Answer from the drawing. Dimensions are ordinates in mm from the lowest x, y and z of the part. A direction names the side the tool comes from. Give positions to 0.01 mm unless a question says otherwise; leave off trailing zeros. Loops run counter-clockwise (first coordinate to the right, second up) from the corner with the lowest first, then second, coordinate; pieces in that order, holes last. Notation, with made-up numbers: (35, 29) - (41, 29) arc R8 ccw to (41, 38) - close; hole circle Ø11 at (74.25, -18). An arc over 180 degrees is marked (long way). One line per question, with ' | ' between items. Start each with the question number.
1. Section C-C (x = 5) is taken. Determine the outline of the cut face in (y, z), plus the area to 4 significant figures.
2. For a pull along X with two mould halves and no side action, classify the marked faces 3, 4 and 5 as released by +X, released by -X, zero draft, split by the parting line, or undercut.
3. Section D-D (x = 7.75) is taken. Determine the outline of the cut face in (y, z).
4. Which of the six approach directions +Z, -Z, +X, -X, +Y, -Y give full straight-line access (tool end or side, diameter ignored) to the marked faces 1 and 2?
5. Each of these flat-tipped pins is pushed along its axis until it touches: pin 1 (1 mm diameter, centred on x = 7.5, z = 0.5, fed in from -Y); pin 2 (1.2 mm diameter, centred on x = 4.5, z = 1, fed in from -Y). Where does it stop, or does it pass through?
6. Section A-A (y = 3.25) is taken. Determine the outline of the cut face in (x, z).
7. Find the intervals of material crossed by line 1 (X direction, y = 3.75, z = 2.05); line 2 (Y direction, x = 3.25, z = 2.1); line 3 (Y direction, x = 9.25, z = 2.2), in increasing order.
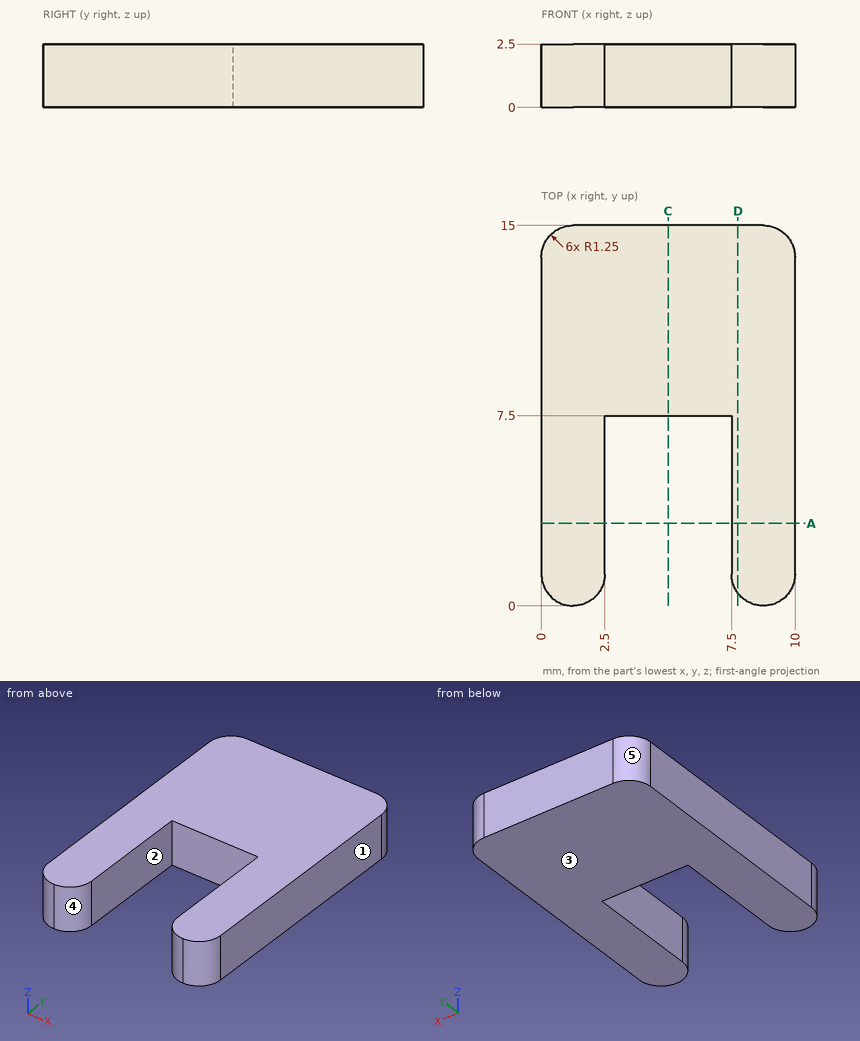
Conclusion:
1) outline: (7.5, 0) - (15, 0) - (15, 2.5) - (7.5, 2.5) - close | area: 18.75 mm²
2) face 3: zero draft | face 4: undercut | face 5: released by -X
3) outline: (0.5, 0) - (15, 0) - (15, 2.5) - (0.5, 2.5) - close
4) face 1: +Z, -Z, +X, +Y, -Y | face 2: +Z, -Z, -Y
5) pin 1: y = 0.25 | pin 2: y = 7.5
6) outline: (0, 0) - (2.5, 0) - (2.5, 2.5) - (0, 2.5) - close; (7.5, 0) - (10, 0) - (10, 2.5) - (7.5, 2.5) - close
7) line 1: 0 to 2.5, 7.5 to 10 | line 2: 7.5 to 15 | line 3: 0.1 to 14.9
